from build123d import *

# Parameters (mm, degrees)
SKETCH1_R           = 5.25
SKETCH1_R_2         = 2.5
SKETCH1_R_3         = 3.225
BOSS_EXTRUDE1_DEPTH = 5


with BuildPart() as part:
    # Sketch1 → Boss-Extrude1 (new body)
    with BuildSketch(Plane(origin=(0, 0, 0), x_dir=(1, 0, 0), z_dir=(0, 1, 0))):
        with BuildLine():
            ThreePointArc((4, 0), (1.171572875, -1.171572875), (0, -4))
            Line((0, -4), (0, -46))
            ThreePointArc((0, -46), (1.171572875, -48.828427125), (4, -50))
            Line((4, -50), (16, -50))
            ThreePointArc((16, -50), (18.828427125, -48.828427125), (20, -46))
            Line((20, -46), (20, -44))
            ThreePointArc((20, -44), (21.171572875, -41.171572875), (24, -40))
            Line((24, -40), (71, -40))
            ThreePointArc((71, -40), (73.828427125, -41.171572875), (75, -44))
            Line((75, -44), (75, -46))
            ThreePointArc((75, -46), (76.171572875, -48.828427125), (79, -50))
            Line((79, -50), (91, -50))
            ThreePointArc((91, -50), (93.828427125, -48.828427125), (95, -46))
            Line((95, -46), (95, -34))
            ThreePointArc((95, -34), (93.828427125, -31.171572875), (91, -30))
            Line((91, -30), (72.250853642, -30))
            ThreePointArc((72.250853642, -30), (71.625426821, -30.005588428), (71, -30))
            ThreePointArc((71, -30), (53.160847909, -24.738723573), (40.535736829, -11.081383158))
            ThreePointArc((40.535736829, -11.081383158), (39.799078859, -10.291604015), (38.759183115, -10))
            Line((38.759183115, -10), (22, -10))
            ThreePointArc((22, -10), (20.585786438, -9.414213562), (20, -8))
            Line((20, -8), (20, -4))
            ThreePointArc((20, -4), (18.828427125, -1.171572875), (16, 0))
            Line((16, 0), (4, 0))
        make_face()
        with Locations(Location((10, -40, 0), (0, 0, 270))):
            Circle(SKETCH1_R, mode=Mode.SUBTRACT)
        with Locations(Location((85, -40, 0), (0, 0, 270))):
            Circle(SKETCH1_R, mode=Mode.SUBTRACT)
        with Locations(Location((35, -25, 0), (0, 0, 270))):
            Circle(SKETCH1_R_2, mode=Mode.SUBTRACT)
        with Locations(Location((10, -10, 0), (0, 0, 270))):
            Circle(SKETCH1_R_3, mode=Mode.SUBTRACT)
    extrude(amount=BOSS_EXTRUDE1_DEPTH)


solid = part.part
The listing builds one solid part. Answer for the finished solid, in the listing's coordinates (mm). A direction names the side the tool comes from. Give positions to 0.01 mm unless a question says otherwise; leave off trailing zeros. Write each loop counter-clockwise with the first axis right and the second up, starting at its lowest first coordinate (ties: lowest second). Pieces come first, ordered by that corner, then holes. Notation, with made-up numbers: (-7.5, 38.5) - (7.5, 38.5) arc R19 ccw to (7.5, 59.5) - close; hole circle Ø2 at (23, 72). An arc over 180 degrees is marked (long way). Use a Markdown table: item, result.
1. Section C-C on x = 10 is taken. Write down the section's boundary in (y, z) (3 decimals).
Values follow:
| item | result |
|---|---|
| outline | (0, 0) - (5, 0) - (5, 6.775) - (0, 6.775) - close; (0, 13.225) - (5, 13.225) - (5, 34.75) - (0, 34.75) - close; (0, 45.25) - (5, 45.25) - (5, 50) - (0, 50) - close |
2. Section A-A on x = 35 is taken. Write down the section's boundary in (y, z), plus the area to 3 significant figures.
Values follow:
| item | result |
|---|---|
| outline | (0, 10) - (5, 10) - (5, 22.5) - (0, 22.5) - close; (0, 27.5) - (5, 27.5) - (5, 40) - (0, 40) - close |
| area | 125 mm² |
3. Each of these flat-tipped pins is pushed along its axis until it touches: P1, Ø1.5, axis at x = 81.5, y = 1.5, coming from the -Z side; P2, Ø3, axis at x = 51, y = 3, coming from the -Z side; P3, Ø2, axis at y = 2.5, z = 6.5, coming from the +X side. Where does it stop, or does it pass through?
Values follow:
| item | result |
|---|---|
| P1 | stops at z = 30 |
| P2 | stops at z = 22.13 |
| P3 | stops at x = 20 |
4. A tool of negligible diameter and unlimited length cuts with its end or side. For faces 4 (the cylindrical face through (93.797, 2.465, 48.859)), 5 (the flat face through (20, 2, 6)), 6 (the cylindrical face through (18.797, 2.465, 48.859)), from which of +Z, -Z, +X, -X, +Y, -Y can it reach the whole face along a straight path? Write none if from no direction.
Values follow:
| item | result |
|---|---|
| face 4 | +Z, +X, +Y, -Y |
| face 5 | -Z, +X, +Y, -Y |
| face 6 | +Z, +Y, -Y |
5. For a pull along X with two mould halves and no side action, classify faces 1 (the flat face through (47, 2, 40)), 2 (the flat face through (95, 2, 40)), 3 (the flat face through (0, 2, 25)) as released by +X, released by -X, zero draft, split by the parting line, or undercut.
Values follow:
| item | result |
|---|---|
| face 1 | undercut |
| face 2 | released by +X |
| face 3 | released by -X |
6. Find the intervals of material crossed by probe 1 along X at (y, z) = (4.05, 38); probe 2 along X at (y, z) = (1.35, 42); probe 3 along X at (y, z) = (3.45, 25), in increasing order. Write a range as from..to.
Values follow:
| item | result |
|---|---|
| probe 1 | x = 0..5.15, 14.85..80.15, 89.85..95 |
| probe 2 | x = 0..5.15, 14.85..20.54, 74.46..80.15, 89.85..95 |
| probe 3 | x = 0..32.5, 37.5..53.59 |
7. Section D-D on z = 38.5 is taken. Write down the section's boundary in (x, y), plus the area to 3 significant figures.
Values follow:
| item | result |
|---|---|
| outline | (0, 0) - (4.97, 0) - (4.97, 5) - (0, 5) - close; (15.03, 0) - (79.97, 0) - (79.97, 5) - (15.03, 5) - close; (90.03, 0) - (95, 0) - (95, 5) - (90.03, 5) - close |
| area | 374 mm² |
8. Section B-B on y = 1.2 is taken. Write down the section's boundary in (x, z) (3 decimals).
Values follow:
| item | result |
|---|---|
| outline | (0, 4) arc R4 ccw to (4, 0) - (16, 0) arc R4 ccw to (20, 4) - (20, 8) arc R2 cw to (22, 10) - (38.759, 10) arc R2 ccw to (40.536, 11.081) arc R35 cw to (71, 30) arc R35 cw to (72.251, 30) - (91, 30) arc R4 ccw to (95, 34) - (95, 46) arc R4 ccw to (91, 50) - (79, 50) arc R4 ccw to (75, 46) - (75, 44) arc R4 cw to (71, 40) - (24, 40) arc R4 cw to (20, 44) - (20, 46) arc R4 ccw to (16, 50) - (4, 50) arc R4 ccw to (0, 46) - close; hole circle Ø10.5 at (10, 40); hole circle Ø6.45 at (10, 10); hole circle Ø5 at (35, 25); hole circle Ø10.5 at (85, 40) |
